from build123d import *

# Parameters (mm, degrees)
F1_DEPTH = 63.5
F3_R     = 1.5875
F4_DEPTH = 6.35
F2_R     = 3.175
F5_DEPTH = 6.35
F6_DEPTH = 6.35


# Not quite as in the source:
# - a feature names something its author has since deleted; it is built from what else it names


with BuildPart() as f1:
    # F0 (on Front) → F1 (new body, symmetric)
    with BuildSketch(Plane.XZ):
        Polygon((38.1, 3.175), (31.75, 3.175), (-31.75, 3.175), (-38.1, 3.175), (-38.1, -22.225), (-19.05, -22.225), (-19.05, -15.875), (-31.75, -15.875), (-31.75, -3.175), (31.75, -3.175), (31.75, -15.875), (19.05, -15.875), (19.05, -22.225), (38.1, -22.225), align=None)
    extrude(amount=F1_DEPTH, both=True)

    # F3 (on face) → F4 (cut)
    with BuildSketch(Plane.YZ.offset(38.1)):
        with Locations((-57.15, -9.525)):
            Circle(F3_R)
        with Locations((-50.8, -9.525)):
            Circle(F3_R)
        with Locations((-44.45, -9.525)):
            Circle(F3_R)
        with Locations((-38.1, -9.525)):
            Circle(F3_R)
        with Locations((-31.75, -9.525)):
            Circle(F3_R)
        with Locations((-25.4, -9.525)):
            Circle(F3_R)
        with Locations((-19.05, -9.525)):
            Circle(F3_R)
        with Locations((-12.7, -9.525)):
            Circle(F3_R)
        with Locations((-6.35, -9.525)):
            Circle(F3_R)
        with Locations((0, -9.525)):
            Circle(F3_R)
        with Locations((6.35, -9.525)):
            Circle(F3_R)
    extrude(amount=-F4_DEPTH, mode=Mode.SUBTRACT)

    # F2 (on face) → F5 (cut)
    with BuildSketch(Plane.XY.offset(3.175)):
        with Locations((0, 11.2886031434)):
            Circle(F2_R)
        with Locations((0, -1.4113968566)):
            Circle(F2_R)
        with Locations((0, -14.1113968566)):
            Circle(F2_R)
    extrude(amount=-F5_DEPTH, mode=Mode.SUBTRACT)

    # F3 (on face) → F6 (cut)
    with BuildSketch(Plane.YZ.offset(38.1)):
        with Locations((12.7, -9.525)):
            Circle(F3_R)
        with Locations((19.05, -9.525)):
            Circle(F3_R)
        with Locations((25.4, -9.525)):
            Circle(F3_R)
        with Locations((31.75, -9.525)):
            Circle(F3_R)
        with Locations((38.1, -9.525)):
            Circle(F3_R)
        with Locations((44.45, -9.525)):
            Circle(F3_R)
        with Locations((50.8, -9.525)):
            Circle(F3_R)
        with Locations((57.15, -9.525)):
            Circle(F3_R)
    extrude(amount=-F6_DEPTH, mode=Mode.SUBTRACT)


solid = f1.part
Design review of the part built by this model. Coordinates are the model's own, in mm. A direction names the side the tool comes from. Round coordinates to 2 decimals unless told otherwise and drop trailing zeros. Write each loop counter-clockwise with the first axis right and the second up, starting at its lowest first coordinate (ties: lowest second). Pieces come first, ordered by that corner, then holes.
Item 1: For pin 1 Ø3 at (y, z) = (57.15, -9.525) entering from +X; pin 2 Ø5 at (y, z) = (-44.45, -9.525) entering from +X, all flat-tipped, find the tip position at first contact; note any pin that passes through.
Item 2: Consider section C-C on x = 26. Give the boundary of the cut face in (y, z) (3 decimals).
Item 3: Consider section D-D on y = 54. Give the boundary of the cut face in (x, z) (3 decimals), and give its area (3 significant figures).
Item 4: Wall thickness on L1, parallel to Z at x = 33.5, y = -51 (3 decimals); L2, parallel to Z at x = 31, y = 34 (3 decimals); L3, parallel to X at y = 34.5, z = -16: over which ranges is each line inside the solid? List them lowest first.
Item 5: Consider section B-B on z = -20.25. Give the boundary of the cut face in (x, y).
Item 6: Draft analysis for pull direction Z (two halves, no side actions). For faces 6 (the flat face through (-8, -1, 3.175)), 7 (the cylindrical face through (34.969, -26.986, -9.455)), 8 (the flat face through (19.05, -1, -19)), state which applies: released by +Z, released by -Z, zero draft, split by the parting line, or undercut.
Item 7: For faces 1 (the flat face through (31.75, -1, -8)), 2 (the flat face through (-29, -1, -22.225)), 3 (the cylindrical face through (34.969, -46.036, -9.455)), 4 (the flat face through (-38.1, -1, -9)), 5 (the flat face through (-19.05, -1, -19)), list the 3-axis set-ups (+Z, -Z, +X, -X, +Y, -Y) from which the entire face can be reached by the end or side of a thin tool; tool diameter is ignored.
Check values:
1. pin 1: stops at x = -31.75
1. pin 2: stops at x = 38.1
2. outline: (-63.5, -22.225) - (63.5, -22.225) - (63.5, -15.875) - (-63.5, -15.875) - close; (-63.5, -3.175) - (63.5, -3.175) - (63.5, 3.175) - (-63.5, 3.175) - close
3. outline: (-38.1, -22.225) - (-19.05, -22.225) - (-19.05, -15.875) - (-31.75, -15.875) - (-31.75, -3.175) - (31.75, -3.175) - (31.75, -15.875) - (19.05, -15.875) - (19.05, -22.225) - (38.1, -22.225) - (38.1, 3.175) - (-38.1, 3.175) - close
3. area: 887 mm2
4. L1: z = -22.225 to -11.1, -7.95 to 3.175
4. L2: z = -22.225 to -15.875, -3.175 to 3.175
4. L3: x = -38.1 to -19.05, 19.05 to 38.1
5. outline: (-38.1, -63.5) - (-19.05, -63.5) - (-19.05, 63.5) - (-38.1, 63.5) - close; (19.05, -63.5) - (38.1, -63.5) - (38.1, 63.5) - (19.05, 63.5) - close
6. face 6: released by +Z
6. face 7: undercut
6. face 8: zero draft
7. face 1: +Y, -Y
7. face 2: -Z, +X, -X, +Y, -Y
7. face 3: +X
7. face 4: +Z, -Z, -X, +Y, -Y
7. face 5: -Z, +Y, -Y
